Autodesk Inventor part; units mm, degrees
ref_plane "YZ Plane" through (0, 0, 0) normal (1, 0, 0) x (0, 1, 0)
ref_plane "XZ Plane" through (0, 0, 0) normal (0, 1, 0) x (-1, 0, 0)
ref_plane "XY Plane" through (0, 0, 0) normal (0, 0, 1) x (1, 0, 0)
sketch "Szkic1" plane through (0, 0, 0) normal (0, 0, 1) x (1, 0, 0)
  line L0 (-40, -27.5) -> (40, -27.5)
  line L1 (40, -27.5) -> (40, 27.5)
  line L2 (40, 27.5) -> (-40, 27.5)
  line L3 (-40, 27.5) -> (-40, -27.5)
  line L4 (-40, -27.5) -> (40, 27.5) construction
  line L5 (40, -27.5) -> (-40, 27.5) construction
  point P0 (0, 0)
  dimension "d0" = 80
  dimension "d1" = 55
extrude "Wyciągnięcie proste1" add sketch "Szkic1" along normal blind 20
sketch "Szkic2" plane through (0, 0, 0) normal (0, 1, 0) x (-1, 0, 0)
  line L0 (39, 0) -> (-11, 0)
  line L1 (-11, 0) -> (-11, -20)
  line L2 (-11, -20) -> (39, -20)
  line L3 (39, -20) -> (39, 0)
  line L4 (40, 0) -> (40, 20)
  line L5 (40, 0) -> (-40, 0)
  point P0 (0, 0)
  dimension "d4" = 50
  dimension "d5" = 20
  dimension "d6" = 1
extrude "Wyciągnięcie proste2" add sketch "Szkic2" along normal mid plane 52
sketch "Szkic3" plane through (0, -26, 0) normal (0, -1, 0) x (1, 0, 0)
  line L0 (11, -20) -> (-39, -20)
  line L1 (-37, -20) -> (-35, -20)
  line L2 (-35, -20) -> (-35, -5)
  line L3 (-35, -5) -> (-37, -5)
  line L4 (-37, -5) -> (-37, -20)
  line L5 (-39, 0) -> (-39, -20)
  line L6 (-33, -20) -> (-31, -20)
  line L7 (-31, -20) -> (-31, -5)
  line L8 (-31, -5) -> (-33, -5)
  line L9 (-33, -5) -> (-33, -20)
  line L10 (-29, -20) -> (-27, -20)
  line L11 (-27, -20) -> (-27, -5)
  line L12 (-27, -5) -> (-29, -5)
  line L13 (-29, -5) -> (-29, -20)
  line L14 (-25, -20) -> (-23, -20)
  line L15 (-23, -20) -> (-23, -5)
  line L16 (-23, -5) -> (-25, -5)
  line L17 (-25, -5) -> (-25, -20)
  line L18 (-21, -20) -> (-19, -20)
  line L19 (-19, -20) -> (-19, -5)
  line L20 (-19, -5) -> (-21, -5)
  line L21 (-21, -5) -> (-21, -20)
  line L22 (-17, -20) -> (-15, -20)
  line L23 (-15, -20) -> (-15, -5)
  line L24 (-15, -5) -> (-17, -5)
  line L25 (-17, -5) -> (-17, -20)
  line L26 (-13, -20) -> (-11, -20)
  line L27 (-11, -20) -> (-11, -5)
  line L28 (-11, -5) -> (-13, -5)
  line L29 (-13, -5) -> (-13, -20)
  line L30 (-9, -20) -> (-7, -20)
  line L31 (-7, -20) -> (-7, -5)
  line L32 (-7, -5) -> (-9, -5)
  line L33 (-9, -5) -> (-9, -20)
  line L34 (-5, -20) -> (-3, -20)
  line L35 (-3, -20) -> (-3, -5)
  line L36 (-3, -5) -> (-5, -5)
  line L37 (-5, -5) -> (-5, -20)
  line L38 (-1, -20) -> (1, -20)
  line L39 (1, -20) -> (1, -5)
  line L40 (1, -5) -> (-1, -5)
  line L41 (-1, -5) -> (-1, -20)
  line L42 (3, -20) -> (5, -20)
  line L43 (5, -20) -> (5, -5)
  line L44 (5, -5) -> (3, -5)
  line L45 (3, -5) -> (3, -20)
  line L46 (7, -20) -> (9, -20)
  line L47 (9, -20) -> (9, -5)
  line L48 (9, -5) -> (7, -5)
  line L49 (7, -5) -> (7, -20)
  point P0 (0, 0)
  dimension "d9" = 2
  dimension "d10" = 15
  dimension "d11" = 2
  dimension "d14" = 4
extrude "Wyciągnięcie proste3" cut sketch "Szkic3" against normal blind 52
properties part number "stepper_driver"
Part model, mm, in its own coordinate system. A direction names the side the tool comes from. Coordinates: 2 decimals unless noted, no trailing zeros. Loops run counter-clockwise (first coordinate to the right, second up) from the corner with the lowest first, then second, coordinate; pieces in that order, holes last. Notation, with made-up numbers: (-14.75, -26) -> (38.25, -26) arc R9 ccw to (38.25, -11) -> close; hole circle Ø10 at (-2.5, 15.25). An arc over 180 degrees is marked (long way). Use a Markdown table: item, result. Add a question column.
Item 1: Band-saw the part on C-C on x = 19. Write the cut outline in (y, z), plus the area to 3 significant figures.
Item 2: Pull direction X, two halves, no side cores. Call faces 1 (the flat face through (11, 0, -10)), 2 (the flat face through (-9, 0, -12)), 3 (the flat face through (-40, 0, 10)), 4 (the flat face through (-22, 0, -20)): +X half, -X half, draft (parallel to the pull), parting line (faces both ways), or undercut.
Item 3: Band-saw the part on B-B on x = -12. Write the cut outline in (y, z).
Item 4: Band-saw the part on A-A on z = -11.5. Give the number of separate pieces and of enclosed holes in the cut face, plus the area to 3 significant figures.
Item 5: Probe probe 1 along Z at (x, y) = (32.5, -14); probe 2 along Z at (x, y) = (-27.5, -2); probe 3 along Y at (x, z) = (-1.5, -9). List the from-to ranges inside material, lowest first.
Item 6: Which spindle directions (+Z, -Z, +X, -X, +Y, -Y) get a long thin tool onto all of the face, cutting with end or side? Do faces 5 (the flat face through (-14, 0, -20)), 6 (the flat face through (-20, 0, -5)). Say none if no direction does.
Item 7: Flat gauge pins, fed straight in: P1, Ø4, axis at x = -17.5, z = -7, coming from the -Y side; P2, Ø4, axis at y = 15.5, z = -11.5, coming from the +X side; P3, Ø1.6, axis at x = -24.5, y = -8.5, coming from the -Z side; P4, Ø1, axis at x = -8, y = -4, coming from the -Z side. Where does each tip first touch, or does it go through?
Geometry says:
| question | item | result |
|---|---|---|
| 1 | outline | (-27.5, 0) -> (27.5, 0) -> (27.5, 20) -> (-27.5, 20) -> close |
| 1 | area | 1,100 mm² |
| 2 | face 1 | +X half |
| 2 | face 2 | undercut |
| 2 | face 3 | -X half |
| 2 | face 4 | draft |
| 3 | outline | (-27.5, 0) -> (-26, 0) -> (-26, -5) -> (26, -5) -> (26, 0) -> (27.5, 0) -> (27.5, 20) -> (-27.5, 20) -> close |
| 4 | separate pieces | 13 |
| 4 | enclosed holes | 0 |
| 4 | area | 1,350 mm² |
| 5 | probe 1 | 0 to 20 |
| 5 | probe 2 | -5 to 20 |
| 5 | probe 3 | -26 to 26 |
| 6 | face 5 | -Z, +X, -X, +Y, -Y |
| 6 | face 6 | -Z, +Y, -Y |
| 7 | P1 | y = -26 |
| 7 | P2 | x = 11 |
| 7 | P3 | z = -20 |
| 7 | P4 | z = -5 |
